Input: part model. Units: mm. Frame: model coordinates. A direction names the side the tool comes from. Give positions to 0.01 mm unless a question says otherwise; leave off trailing zeros. Write each loop counter-clockwise with the first axis right and the second up, starting at its lowest first coordinate (ties: lowest second). Pieces come first, ordered by that corner, then holes.
```python
from build123d import *

# Parameters (mm, degrees)
SKETCH1_W           = 58
SKETCH1_H           = 35.5
SKETCH1_R           = 1.5
BOSS_EXTRUDE1_DEPTH = 1.5
SKETCH2_W           = 58
SKETCH2_H           = 9.9
SKETCH2_R           = 1.5
BOSS_EXTRUDE3_DEPTH = 1.5
FILLET1_R           = 2.2
SKETCH2_3_W         = 10
SKETCH2_3_H         = 4.7
BOSS_EXTRUDE4_DEPTH = 3
CHAMFER1_SIZE       = 3
FILLET2_R           = 2


# Some blends are built 0.0001 mm under size
with BuildPart() as part:
    # Sketch1 → Boss-Extrude1 (new body)
    with BuildSketch(Plane(origin=(0, 0, 0), x_dir=(1, 0, 0), z_dir=(0, 1, 0))):
        Rectangle(SKETCH1_W, SKETCH1_H)
        with Locations(Location((-25.5, 14.25, 0), (0, 0, 270))):
            Circle(SKETCH1_R, mode=Mode.SUBTRACT)
        with Locations(Location((25.5, 14.25, 0), (0, 0, 90))):
            Circle(SKETCH1_R, mode=Mode.SUBTRACT)
    extrude(amount=BOSS_EXTRUDE1_DEPTH)

    # Sketch2 → Boss-Extrude3 (add)
    with BuildSketch(Plane(origin=(0, 1.5, 0), x_dir=(1, 0, 0), z_dir=(0, 1, 0))):
        with Locations((0, 12.8)):
            Rectangle(SKETCH2_W, SKETCH2_H)
        with Locations(Location((-25.5, 14.25, 0), (0, 0, 270))):
            Circle(SKETCH2_R, mode=Mode.SUBTRACT)
        with Locations(Location((25.5, 14.25, 0), (0, 0, 90))):
            Circle(SKETCH2_R, mode=Mode.SUBTRACT)
    extrude(amount=BOSS_EXTRUDE3_DEPTH)

    # Fillet1
    # the kernel refuses this fillet: 2.2 mm, written as the material it adds along each edge
    with BuildSketch(Plane(origin=(-29, 1.5, -7.85), x_dir=(0, 0, 1), z_dir=(1, 0, 0))) as fillet1_piece_1:
        with BuildLine():
            CenterArc((2.085665361, -2.2), FILLET1_R, 90, 71.446995465)
            Line((0, -1.5), (-0.041713307, -1.486))
            ThreePointArc((-0.041713307, -1.486), (-0.044, -0.75), (-0.044, 0))
            Line((-0.044, 0), (0, 0.044))
            Line((0, 0.044), (2.085665361, 0.044))
            Line((2.085665361, 0.044), (2.085665361, 0))
        make_face()
    extrude(amount=58)

    # Sketch2<3> → Boss-Extrude4 (add)
    with BuildSketch(Plane(origin=(0, 1.5, 0), x_dir=(1, 0, 0), z_dir=(0, 1, 0))):
        with Locations((0, -20.1)):
            Rectangle(SKETCH2_3_W, SKETCH2_3_H)
        with Locations((0, -15.4)):
            Rectangle(SKETCH2_3_W, SKETCH2_3_H)
    extrude(amount=BOSS_EXTRUDE4_DEPTH)

    # Chamfer1
    chamfer1_edges = [part.edges().sort_by_distance(p)[0] for p in [
        (0, 4.5, 13.05),
        (0, 4.5, 22.45),
    ]]
    chamfer(chamfer1_edges, length=CHAMFER1_SIZE - 0.0001)  # a hair under: the kernel refuses the full size

    # Fillet2
    fillet2_edges = [part.edges().sort_by_distance(p)[0] for p in [
        (-29, 1.5, -17.75),
        (29, 1.5, -17.75),
    ]]
    fillet(fillet2_edges, radius=FILLET2_R)


solid = part.part
```
Q1. Section D-D, the plane z = -3. Return the cut outline in (x, y), then the cut area to 3 significant figures.
Q2. Section C-C, the plane x = -14.5. Return the cut outline in (y, z), then the cut area to 3 significant figures.
Q3. Section B-B, the plane z = -14.25. Return the cut outline in (x, y), then the cut area to 3 significant figures.
Q4. Section A-A, the plane x = -25.5. Return the cut outline in (y, z).
Q5. Mould query, pull axis X, two halves, no side actions, for faces 4 (the cylindrical face through (24.49, 1.48, -13.14)), 5 (the flat face through (0, 4.5, 18)), 6 (the flat face through (29, 1, -2)). Classes: +X half, -X half, draft (parallel to the pull), parting line (faces both ways), or undercut.
Q6. Material intervals for line 1 along X through (y, z) = (0.75, -14.25); line 2 along Z through (x, y) = (25.5, 0.7); line 3 along Z through (x, y) = (-7, 1.4), sorted ascending.
Q7. Pin query (flat end, axial travel): pin 1 (5 mm diameter, centred on x = -5.5, z = -13.5, fed in from +Y); pin 2 (1.5 mm diameter, centred on y = 3, z = 19.5, fed in from +X); pin 3 (12 mm diameter, centred on x = -9.5, z = 8, fed in from +Y). Return the tip coordinate at first contact, or that it passes through.
Q8. Access query for faces 1 (the flat face through (5, 3, 18)), 2 (the flat face through (0, 1.5, 20)), 3 (the flat face through (-0.07, 2.98, 14.53)). Directions: +Z, -Z, +X, -X, +Y, -Y. A direction counts if a zero-diameter tool reaches every point of the face in a straight line with its end or side. Return the directions, or none.
Solutions:
1. outline: (-29, 0) - (29, 0) - (29, 1.5) - (-29, 1.5) - close
1. area: 87.0 mm2
2. outline: (0, -17.75) - (3, -17.75) - (3, -7.85) arc R2.2 cw to (1.5, -5.76) - (1.5, 17.75) - (0, 17.75) - close
2. area: 68.9 mm2
3. outline: (-29, 0) - (-27, 0) - (-27, 3) - (-29, 3) - close; (-24, 0) - (24, 0) - (24, 3) - (-24, 3) - close; (27, 0) - (29, 0) - (29, 3) - (27, 3) - close
3. area: 156 mm2
4. outline: (0, -17.75) - (3, -17.75) - (3, -15.75) - (0, -15.75) - close; (0, -12.75) - (3, -12.75) - (3, -7.85) arc R2.2 cw to (1.5, -5.76) - (1.5, 17.75) - (0, 17.75) - close
5. face 4: undercut
5. face 5: draft
5. face 6: +X half
6. line 1: x = -29 to -27, -24 to 24, 27 to 29
6. line 2: z = -17.75 to -15.75, -12.75 to 17.75
6. line 3: z = -17.75 to 17.75
7. pin 1: stops at y = 3
7. pin 2: stops at x = 5
7. pin 3: stops at y = 1.5
8. face 1: +Z, +X, +Y
8. face 2: +Z, +X, -X, -Y
8. face 3: +X, -X, +Y
